from build123d import *

# Parameters (mm, degrees)
SKETCH1_W           = 500
SKETCH1_H           = 800
SKETCH1_R           = 1.905
SKETCH1_R_2         = 3.175
SKETCH1_W_2         = 347.6
SKETCH1_H_2         = 457.2
BOSS_EXTRUDE1_DEPTH = 7.62


with BuildPart() as part:
    # Sketch1 → Boss-Extrude1 (new body)
    with BuildSketch(Plane.XY):
        Rectangle(SKETCH1_W, SKETCH1_H)
        with Locations((136.462, -125.68)):
            Circle(SKETCH1_R, mode=Mode.SUBTRACT)
        with Locations((211.138, -125.68)):
            Circle(SKETCH1_R, mode=Mode.SUBTRACT)
        with Locations((211.138, -174.448)):
            Circle(SKETCH1_R, mode=Mode.SUBTRACT)
        with Locations((136.462, -174.448)):
            Circle(SKETCH1_R, mode=Mode.SUBTRACT)
        with Locations((237.3, -215.85)):
            Circle(SKETCH1_R_2, mode=Mode.SUBTRACT)
        with Locations((110.3, -215.85)):
            Circle(SKETCH1_R_2, mode=Mode.SUBTRACT)
        with Locations((237.3, -253.95)):
            Circle(SKETCH1_R_2, mode=Mode.SUBTRACT)
        with Locations((110.3, -253.95)):
            Circle(SKETCH1_R_2, mode=Mode.SUBTRACT)
        with Locations((0, 133.3)):
            Rectangle(SKETCH1_W_2, SKETCH1_H_2, mode=Mode.SUBTRACT)
        with BuildLine():
            Line((156.274, -128.728), (191.326, -128.728))
            ThreePointArc((191.326, -128.728), (212.662, -150.064), (191.326, -171.4))
            Line((191.326, -171.4), (156.274, -171.4))
            ThreePointArc((156.274, -171.4), (134.938, -150.064), (156.274, -128.728))
        make_face(mode=Mode.SUBTRACT)
        with BuildLine():
            Line((224.6, -241.25), (123, -241.25))
            ThreePointArc((123, -241.25), (116.65, -234.9), (123, -228.55))
            Line((123, -228.55), (224.6, -228.55))
            ThreePointArc((224.6, -228.55), (230.95, -234.9), (224.6, -241.25))
        make_face(mode=Mode.SUBTRACT)
    extrude(amount=BOSS_EXTRUDE1_DEPTH)


solid = part.part
For this review, take the finished solid that the model builds, in its own axes (mm). A direction names the side the tool comes from. Give positions to 0.01 mm unless a question says otherwise; leave off trailing zeros. Loops run counter-clockwise (first coordinate to the right, second up) from the corner with the lowest first, then second, coordinate; pieces in that order, holes last.
Item 1: Tool access review of faces 1 (the cylindrical face through (134.943, -150.533, 3.757)), 2 (the flat face through (-3, -172, 0)): name each direction out of +Z, -Z, +X, -X, +Y, -Y from which nothing blocks a thin tool from reaching the whole face with its end or side.
Item 2: Insertion check: pin 1 (5 mm diameter, centred on x = 211.138, y = -174.448, fed in from +Z). The pin has a flat end and moves straight along its axis. Give the tip position at first contact, or say it passes through.
Item 3: Take a section at A-A, the plane y = 126.5. State the section outline as (x, z) points.
Item 4: Draft analysis for pull direction X (two halves, no side actions). For faces 3 (the cylindrical face through (212.657, -149.595, 3.757)), 4 (the flat face through (-3, -172, 7.62)), state which applies: +X half, -X half, draft (parallel to the pull), parting line (faces both ways), or undercut.
Item 5: For line 1 along X through (y, z) = (-215.85, 3.5) (3 decimals); line 2 along Y through (x, z) = (237.3, 4) (3 decimals); line 3 along X through (y, z) = (215.5, 7.5), list the stretches that pass through material, from the lowest coordinate up.
Item 6: Take a section at C-C, the plane z = 4.25. Give the number of separate pieces and of enclosed holes in the cut face, and give its area (3 significant figures).
Item 7: Take a section at B-B, the plane x = -55. State the section outline as (y, z) points.
Calculated:
1. face 1: +Z, -Z
1. face 2: -Z, +X, -X, +Y, -Y
2. pin 1: stops at z = 7.62
3. outline: (-250, 0) - (-173.8, 0) - (-173.8, 7.62) - (-250, 7.62) - close; (173.8, 0) - (250, 0) - (250, 7.62) - (173.8, 7.62) - close
4. face 3: undercut
4. face 4: draft
5. line 1: x = -250 to 107.125, 113.475 to 234.125, 240.475 to 250
5. line 2: y = -400 to -257.125, -250.775 to -219.025, -212.675 to 400
5. line 3: x = -250 to -173.8, 173.8 to 250
6. separate pieces: 1
6. enclosed holes: 11
6. area: 237,000 mm2
7. outline: (-400, 0) - (-95.3, 0) - (-95.3, 7.62) - (-400, 7.62) - close; (361.9, 0) - (400, 0) - (400, 7.62) - (361.9, 7.62) - close
